from build123d import *

# Parameters (mm, degrees)
R_P_TITION_CIRCULAIRE7_COUNT = 4


with BuildPart() as part:
    # Esquisse1 → Révolution1 (revolve)
    with BuildSketch(Plane(origin=(0, 0, 0), x_dir=(1, 0, 0), z_dir=(0, 1, 0))):
        Polygon((-18.460120385, 0), (-18.460120385, 2), (-12.160120385, 2), (-12.160120385, 7), (-8.660120385, 7), (-8.660120385, 17.5), (35.703488783, 17.5), (36.539879615, 15.8), (38.539879615, 15.8), (38.539879615, 8), (39.939879615, 8), (39.939879615, 2), (52.339879615, 2), (52.339879615, 0), align=None)
    revolve(axis=Axis((52.339879615, 0, 0), (-1, 0, 0)))

    # Esquisse4 → Trou taraudé M22 (revolve, cut)
    with BuildSketch(Plane(origin=(38.539879615, 0, -11), x_dir=(0, 0, -1), z_dir=(0, 1, 0))):
        Polygon((0, 0), (0, 5.180688495), (0.8, 4.7), (0.8, 0), align=None)
    trou_taraud_m22 = revolve(axis=Axis((44.889879615, 0, -11), (-1, 0, 0)), mode=Mode.SUBTRACT)

    # Répétition circulaire7: Trou taraudé M22 ×4 about axis
    r_p_tition_circulaire7_axis = Axis((0, 0, 0), (1, 0, 0))
    for i in range(1, R_P_TITION_CIRCULAIRE7_COUNT):
        add(trou_taraud_m22.rotate(r_p_tition_circulaire7_axis, i * 360 / R_P_TITION_CIRCULAIRE7_COUNT), mode=Mode.SUBTRACT)


solid = part.part
Build history of the part. All positions in model axes, mm. A direction names the side the tool comes from. Coordinates: 2 decimals unless noted, no trailing zeros. Order: outer loops, then holes, each group sorted by start corner. A loop starts at its lowest first (then second) coordinate and runs counter-clockwise, first axis right, second up. Notation, with made-up numbers: (82.25, 25.5) - (105.25, 25.5) arc R22 ccw to (105.25, 45.5) - close; hole circle Ø10 at (43.5, 77.25). An arc over 180 degrees is marked (long way). Write each question's results on one line, items separated by ' | '. Start each with the question number.
Item 1: Flat gauge pins, fed straight in: pin 1 (1 mm diameter, centred on y = 11, z = 0, fed in from -X); pin 2 (1 mm diameter, centred on y = -3, z = -12.5, fed in from +X); pin 3 (3 mm diameter, centred on x = 37, y = 6, fed in from +Z); pin 4 (10 mm diameter, centred on x = 44.5, z = 11, fed in from +Y). Where does each tip first touch, or does it go through?
Item 2: Band-saw the part on B-B on x = 46. Write the cut outline in (y, z).
Item 3: Mould opens along Y. For faces 4 (the face through (33.443, 10.861, -0.006)), 5 (the face through (-10.386, 2.681, -6.466)), 6 (the face through (-18.46, 0, 0)) say: released by +Y, released by -Y, zero draft, split by the parting line, or undercut.
Item 4: Tool access for faces 1 (the face through (39.25, 7.81, 1.73)), 2 (the face through (-8.66, 8, 0)), 3 (the face through (52.34, 0, 0)): list every direction of +Z, -Z, +X, -X, +Y, -Y with a clear straight run to the whole face (end or side of a thin tool).
Item 5: Band-saw the part on A-A on x = 26.5. Write the cut outline in (y, z), and give its area (3 significant figures).
Item 6: Wall check: probe 1 along Y at (x, z) = (29.5, 0); probe 2 along Y at (x, z) = (35.35, -11); probe 3 along X at (y, z) = (-1, 6). Give the ranges that are in metal, low to high. Write a range as [from, to].
Numbers:
1) pin 1: x = -8.66 | pin 2: x = 38.54 | pin 3: z = 16.7 | pin 4: through
2) outline: circle Ø4 at (0, 0)
3) face 4: undercut | face 5: split by the parting line | face 6: zero draft
4) face 1: +X | face 2: -X | face 3: +Z, -Z, +X, +Y, -Y
5) outline: circle Ø35 at (0, 0) | area: 962 mm^2
6) probe 1: [-17.5, 17.5] | probe 2: [-13.61, -0.8], [0.8, 13.61] | probe 3: [-12.16, 39.94]
